The model under review builds one solid part; all positions refer to its coordinate system, in mm. Give positions to 0.01 mm unless a question says otherwise; leave off trailing zeros. Write each loop counter-clockwise with the first axis right and the second up, starting at its lowest first coordinate (ties: lowest second). Pieces come first, ordered by that corner, then holes. Notation, with made-up numbers: M 53.25,-7 L 62.25,-7 A30 cw 62.25,21 Z; hole C 1,67.25 d2. An arc over 180 degrees is marked long. Write each question's results on one line, items separated by ' | '. Start each with the question number.
from build123d import *

# Parameters (mm, degrees)
F1_DEPTH    = 2500
F2_T1_DEPTH = 2500
F3_R        = 3.99999


# Not quite as in the source:
# - a fillet or chamfer that OpenCascade refuses, or shapes differently, is made with other operations: its cross-section is extruded or revolved along the edge and cut away or added
# - a fillet or chamfer is up to 0.001 mm smaller than in the source, because OpenCascade refuses the exact size


with BuildPart() as f1:
    # F0 (on Top) → F1 (new body)
    with BuildSketch(Plane.XY):
        Polygon((-50, -25), (50, -25), (50, 25), (46, 25), (46, -21), (-46, -21), (-46, 25), (-50, 25), align=None)
    extrude(amount=F1_DEPTH)

    # F2: fillet of radius 10 on 2 edges, made by hand

    # F2_s2 → F2_t1 (join)
    with BuildSketch(Plane.XY):
        with BuildLine():
            add(Edge.make_bspline(
                [(46, -11), (46, -21), (36, -21)],
                knots=[0, 0, 0, 1, 1, 1], degree=2, weights=[1, 1, 1]))
            Line((36, -21), (46, -21))
            Line((46, -21), (46, -11))
        make_face()
        with BuildLine():
            add(Edge.make_bspline(
                [(-36, -21), (-46, -21), (-46, -11)],
                knots=[0, 0, 0, 1, 1, 1], degree=2, weights=[1, 1, 1]))
            Line((-46, -11), (-46, -21))
            Line((-46, -21), (-36, -21))
        make_face()
    extrude(amount=F2_T1_DEPTH)

    # F3 (radius 4 in the source; OpenCascade refuses exactly that, so slightly less here)
    f3_edges = [f1.edges().sort_by_distance(p)[0] for p in [
        (-46, 25, 1250),
        (46, 25, 1250),
    ]]
    fillet(f3_edges, radius=F3_R)


solid = f1.part
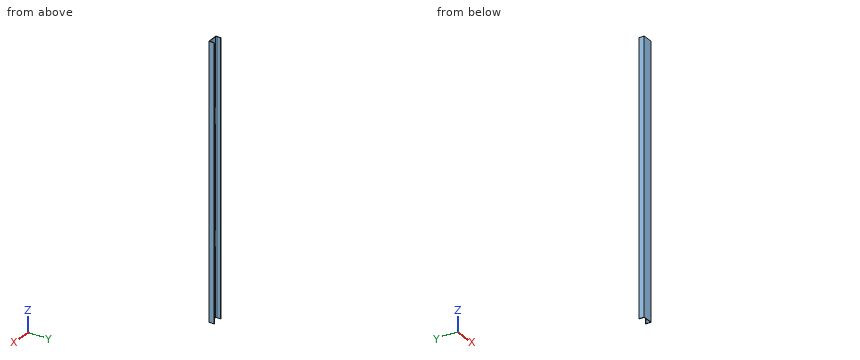
(1) Wall thickness on L1, parallel to X at y = -14, z = 251; L2, parallel to X at y = -1.5, z = 1400; L3, parallel to Y at x = 32, z = 791.5: over which ranges is each line inside the solid? List them lowest first.
(2) Clearance check with a flat-ended pin moving along its axis: P1, Ø8, axis at x = 24, z = 1236, coming from the +Y side. State where the tip first meets the part, or that it passes through.
(3) Add section A-A (x = 1). State the section outline as (y, z) points, then the cut area to 3 significant figures.
Calculated:
1) L1: x = -50 to -45.73, 45.73 to 50 | L2: x = -50 to -46, 46 to 50 | L3: y = -25 to -21
2) P1: stops at y = -21
3) outline: M -25,0 L -21,0 L -21,2500 L -25,2500 Z | area: 10,000 mm²
